Can you work these out from the model? Positions are in its coordinate system, mm. A direction names the side the tool comes from. Give positions to 0.01 mm unless a question says otherwise; leave off trailing zeros. Order: outer loops, then holes, each group sorted by start corner. A loop starts at its lowest first (then second) coordinate and runs counter-clockwise, first axis right, second up. Notation, with made-up numbers: (36, 0.25) -> (56, 0.25) arc R21 cw to (56, 26.25) -> close; hole circle Ø8 at (81.5, 13.5). An arc over 180 degrees is marked (long way). Answer as a JSON object with one key per item and string values.
```python
from build123d import *

# Parameters (mm, degrees)
F_3_8_CLEARANCE_HOLE1_D = 10.0838
CIRPATTERN1_COUNT       = 10
SKETCH5_RX              = 50.8
SKETCH5_RY              = 31.75
CUT_EXTRUDE1_DEPTH      = 2.032
SKETCH6_R               = 0.79375
CUT_EXTRUDE2_DEPTH      = 108.849548557


with BuildPart() as part:
    # Sketch1 → Revolve1 (revolve)
    with BuildSketch(Plane.XY, mode=Mode.PRIVATE) as revolve1_sk:
        Polygon((0, -6.35), (54.8259, -6.35), (54.8259, -3.6576), (58.8899, -3.6576), (58.8899, -6.35), (76.2, -6.35), (76.2, 0), (0, 0), align=None)
    revolve(revolve1_sk.sketch.rotate(Axis((0, 0, 0), (0, -1, 0)), 90), axis=Axis((0, 0, 0), (0, -1, 0)))

    # 3_8 Clearance Hole1 (through all)
    with Locations(Plane(origin=(67.31, 0, 0), x_dir=(0, 0, 1), z_dir=(0, 1, 0))):
        with Locations((0, 0)):
            f_3_8_clearance_hole1 = Hole(F_3_8_CLEARANCE_HOLE1_D / 2)

    # CirPattern1: 3_8 Clearance Hole1 ×10 about axis
    cirpattern1_axis = Axis((0, 0, 0), (0, 1, 0))
    for i in range(1, CIRPATTERN1_COUNT):
        add(f_3_8_clearance_hole1.rotate(cirpattern1_axis, i * 360 / CIRPATTERN1_COUNT), mode=Mode.SUBTRACT)

    # Sketch5 → Cut-Extrude1 (cut)
    with BuildSketch(Plane(origin=(0, 0, 0), x_dir=(1, 0, 0), z_dir=(0, 1, 0))):
        with Locations((0, 0)):
            Ellipse(SKETCH5_RX, SKETCH5_RY)
        with BuildLine():
            Line((-3.302199606, -2.201466404), (-28.702199606, 35.898533596))
            ThreePointArc((-28.702199606, 35.898533596), (-27.601466404, 41.402199606), (-22.097800394, 40.301466404))
            Line((-22.097800394, 40.301466404), (3.302199606, 2.201466404))
            ThreePointArc((3.302199606, 2.201466404), (2.201466404, -3.302199606), (-3.302199606, -2.201466404))
        make_face()
    extrude(amount=-CUT_EXTRUDE1_DEPTH, mode=Mode.SUBTRACT)

    # Sketch6 → Cut-Extrude2 (cut, through all)
    with BuildSketch(Plane(origin=(0, -2.032, 0), x_dir=(1, 0, 0), z_dir=(0, 1, 0))):
        with Locations(Location((13.97, 0, 0), (0, 0, 270))):
            Circle(SKETCH6_R)
        with Locations(Location((20.32, 0, 0), (0, 0, 270))):
            Circle(SKETCH6_R)
        with Locations(Location((26.67, 0, 0), (0, 0, 270))):
            Circle(SKETCH6_R)
        with Locations(Location((12.586535085, -6.061355835, 0), (0, 0, 270))):
            Circle(SKETCH6_R)
        with Locations(Location((18.307687396, -8.816517579, 0), (0, 0, 270))):
            Circle(SKETCH6_R)
        with Locations(Location((24.028839707, -11.571679322, 0), (0, 0, 270))):
            Circle(SKETCH6_R)
        with Locations(Location((8.710152532, -10.92218581, 0), (0, 0, 270))):
            Circle(SKETCH6_R)
        with Locations(Location((12.669312774, -15.886815724, 0), (0, 0, 270))):
            Circle(SKETCH6_R)
        with Locations(Location((16.628473016, -20.851445637, 0), (0, 0, 270))):
            Circle(SKETCH6_R)
        with Locations(Location((3.108617447, -13.619742933, 0), (0, 0, 270))):
            Circle(SKETCH6_R)
        with Locations(Location((4.521625378, -19.810535176, 0), (0, 0, 270))):
            Circle(SKETCH6_R)
        with Locations(Location((5.934633309, -26.001327418, 0), (0, 0, 270))):
            Circle(SKETCH6_R)
        with Locations(Location((-3.108617447, -13.619742933, 0), (0, 0, 270))):
            Circle(SKETCH6_R)
        with Locations(Location((-4.521625378, -19.810535176, 0), (0, 0, 270))):
            Circle(SKETCH6_R)
        with Locations(Location((-5.934633309, -26.001327418, 0), (0, 0, 270))):
            Circle(SKETCH6_R)
        with Locations(Location((-8.710152532, -10.92218581, 0), (0, 0, 270))):
            Circle(SKETCH6_R)
        with Locations(Location((-12.669312774, -15.886815724, 0), (0, 0, 270))):
            Circle(SKETCH6_R)
        with Locations(Location((-16.628473016, -20.851445637, 0), (0, 0, 270))):
            Circle(SKETCH6_R)
        with Locations(Location((-12.586535085, -6.061355835, 0), (0, 0, 270))):
            Circle(SKETCH6_R)
        with Locations(Location((-18.307687396, -8.816517579, 0), (0, 0, 270))):
            Circle(SKETCH6_R)
        with Locations(Location((-24.028839707, -11.571679322, 0), (0, 0, 270))):
            Circle(SKETCH6_R)
        with Locations(Location((-13.97, 0, 0), (0, 0, 270))):
            Circle(SKETCH6_R)
        with Locations(Location((-20.32, 0, 0), (0, 0, 270))):
            Circle(SKETCH6_R)
        with Locations(Location((-26.67, 0, 0), (0, 0, 270))):
            Circle(SKETCH6_R)
        with Locations(Location((-12.586535085, 6.061355835, 0), (0, 0, 270))):
            Circle(SKETCH6_R)
        with Locations(Location((-18.307687396, 8.816517579, 0), (0, 0, 270))):
            Circle(SKETCH6_R)
        with Locations(Location((-24.028839707, 11.571679322, 0), (0, 0, 270))):
            Circle(SKETCH6_R)
        with Locations(Location((-8.710152532, 10.92218581, 0), (0, 0, 270))):
            Circle(SKETCH6_R)
        with Locations(Location((-12.669312774, 15.886815724, 0), (0, 0, 270))):
            Circle(SKETCH6_R)
        with Locations(Location((-16.628473016, 20.851445637, 0), (0, 0, 270))):
            Circle(SKETCH6_R)
        with Locations(Location((-3.108617447, 13.619742933, 0), (0, 0, 270))):
            Circle(SKETCH6_R)
        with Locations(Location((-4.521625378, 19.810535176, 0), (0, 0, 270))):
            Circle(SKETCH6_R)
        with Locations(Location((-5.934633309, 26.001327418, 0), (0, 0, 270))):
            Circle(SKETCH6_R)
        with Locations(Location((3.108617447, 13.619742933, 0), (0, 0, 270))):
            Circle(SKETCH6_R)
        with Locations(Location((4.521625378, 19.810535176, 0), (0, 0, 270))):
            Circle(SKETCH6_R)
        with Locations(Location((5.934633309, 26.001327418, 0), (0, 0, 270))):
            Circle(SKETCH6_R)
        with Locations(Location((8.710152532, 10.92218581, 0), (0, 0, 270))):
            Circle(SKETCH6_R)
        with Locations(Location((12.669312774, 15.886815724, 0), (0, 0, 270))):
            Circle(SKETCH6_R)
        with Locations(Location((16.628473016, 20.851445637, 0), (0, 0, 270))):
            Circle(SKETCH6_R)
        with Locations(Location((12.586535085, 6.061355835, 0), (0, 0, 270))):
            Circle(SKETCH6_R)
        with Locations(Location((18.307687396, 8.816517579, 0), (0, 0, 270))):
            Circle(SKETCH6_R)
        with Locations(Location((24.028839707, 11.571679322, 0), (0, 0, 270))):
            Circle(SKETCH6_R)
    extrude(amount=-CUT_EXTRUDE2_DEPTH, mode=Mode.SUBTRACT)


solid = part.part
```
1. If we section it at D-D on z = -38.1: Please give me the cut outline in (x, y).
Worked answers:
{"outline": "(-65.99, -6.35) -> (-59.28, -6.35) -> (-59.28, 0) -> (-65.99, 0) -> close; (-49.63, -6.35) -> (-44.9, -6.35) -> (-44.9, -3.66) -> (-39.42, -3.66) -> (-39.42, -6.35) -> (39.42, -6.35) -> (39.42, -3.66) -> (44.9, -3.66) -> (44.9, -6.35) -> (49.63, -6.35) -> (49.63, 0) -> (-20.63, 0) -> (-20.63, -2.03) -> (-29.37, -2.03) -> (-29.37, 0) -> (-49.63, 0) -> close; (59.28, -6.35) -> (65.99, -6.35) -> (65.99, 0) -> (59.28, 0) -> close"}
2. Please list where these lines run through material, in increasing order: L1, parallel to X at y = -2, z = 3; L2, parallel to Z at x = -39, y = -6; L3, parallel to Z at x = -45, y = -5.75.
Worked answers:
{"L1": "-76.14 to -71.36, -63.26 to -50.57, 50.57 to 63.26, 71.36 to 76.14", "L2": "-65.46 to -44.13, -38.53 to 38.53, 44.13 to 65.46", "L3": "-61.49 to -37.99, -31.32 to 31.32, 37.99 to 61.49"}
3. If we section it at C-C on y = -4.75: Count the separate pieces of the cut face and the enclosed holes in it, then the cut area to 3 significant figures.
Worked answers:
{"separate pieces": "2", "enclosed holes": "53", "area": "15,900 mm²"}
4. If we section it at A-A on x = -67.31: Please give me the cut outline in (y, z), then the cut area to 3 significant figures.
Worked answers:
{"outline": "(-6.35, -35.72) -> (0, -35.72) -> (0, -5.04) -> (-6.35, -5.04) -> close; (-6.35, 5.04) -> (0, 5.04) -> (0, 35.72) -> (-6.35, 35.72) -> close", "area": "390 mm²"}
5. If we section it at B-B on z = 53: Please give me the cut outline in (x, y), then the cut area to 3 significant figures.
Worked answers:
{"outline": "(-54.75, -6.35) -> (-25.67, -6.35) -> (-25.67, -3.66) -> (-14.03, -3.66) -> (-14.03, -6.35) -> (14.03, -6.35) -> (14.03, -3.66) -> (25.67, -3.66) -> (25.67, -6.35) -> (54.75, -6.35) -> (54.75, 0) -> (-54.75, 0) -> close", "area": "633 mm²"}
6. If we mould it in two halves opening along Z, with no side actions, what happens to faces 1 (the face through (74.388, -3.131, -16.519)), 2 (the face through (-1, 0, 33)), 3 (the face through (-71.56, -3.22, 2.71))? For each: +Z half, -Z half, draft (parallel to the pull), parting line (faces both ways), or undercut.
Worked answers:
{"face 1": "parting line", "face 2": "draft", "face 3": "undercut"}
7. Will these pins go through, and if not, where does the flat tip stop? pin 1 Ø3 at (x, y) = (-5.5, -2.5) entering from +Z; pin 2 Ø2 at (y, z) = (-5, 52.5) entering from -X; pin 3 Ø2 at (x, z) = (-4.52, 19.81) entering from +Y.
Worked answers:
{"pin 1": "z = 76.09", "pin 2": "x = -56.16", "pin 3": "y = -2.03"}
8. For faces 4 (the face through (39, -3.658, -39)), 5 (the face through (71.56, -3.22, -2.71)), 6 (the face through (-26.079, -1.002, -31.964)), which set-ups out of +Z, -Z, +X, -X, +Y, -Y let a thin tool reach every point of the face, with its end or its side?
Worked answers:
{"face 4": "-Y", "face 5": "+Y, -Y", "face 6": "+Y"}
